Design review of the part built by this model. Coordinates are the model's own, in mm. Face numbers are marked on the shaded views. Coordinates: 2 decimals unless noted, no trailing zeros. Loops run counter-clockwise (first coordinate to the right, second up) from the corner with the lowest first, then second, coordinate; pieces in that order, holes last.
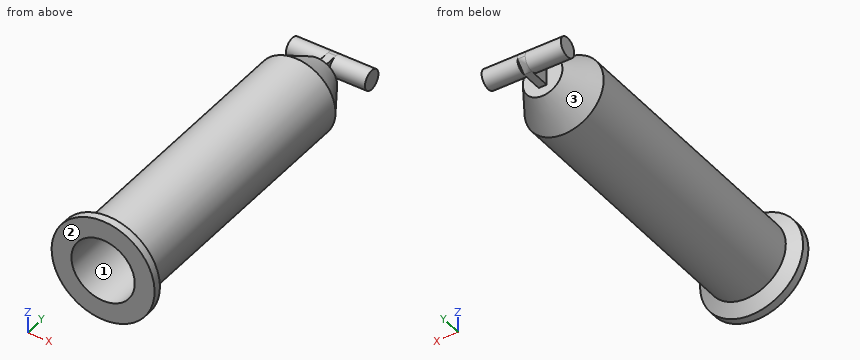
from build123d import *
from build123d.topology import SkipClean

# Parameters (mm, degrees)
SKETCH2_W                = 2
SKETCH2_H                = 5
BOSS_EXTRUDE1_DEPTH      = 8
CUT_EXTRUDE1_DEPTH       = 91.049986119
CUT_EXTRUDE1_DEPTH_BACK  = 91.049986119
SKETCH3_3_R              = 2.5
BOSS_EXTRUDE2_DEPTH      = 9
BOSS_EXTRUDE2_DEPTH_BACK = 11


with BuildPart() as part:
    # Sketch1 → Revolve1 (revolve)
    with BuildSketch(Plane(origin=(0, 0, 0), x_dir=(0, 0, -1), z_dir=(1, 0, 0))):
        Polygon((-10, 4), (-10, 72), (-5, 80), (0, 80), (0, 71.426407547), (-8, 71.426407547), (-8, 0), (-13, 0), (-13, 2), align=None)
    revolve(axis=Axis((0, 80, 0), (0, -1, 0)))

    # Sketch2 → Boss-Extrude1 (add)
    with BuildSketch(Plane(origin=(0, 80, 0), x_dir=(1, 0, 0), z_dir=(0, 1, 0))):
        Rectangle(SKETCH2_W, SKETCH2_H)
    extrude(amount=BOSS_EXTRUDE1_DEPTH)

    # Sketch3 → Cut-Extrude1 (cut, two sides)
    with BuildSketch(Plane.ZY.offset(1)) as cut_extrude1_sk:
        with BuildLine():
            ThreePointArc((-2.2e-08, 88), (1.767766945, 87.267766961), (2.5, 85.5))
            Line((2.5, 85.5), (2.5, 88))
            Line((2.5, 88), (-2.2e-08, 88))
        make_face()
        with BuildLine():
            Line((-2.5, 88), (-2.5, 85.5))
            ThreePointArc((-2.5, 85.5), (-1.767766961, 87.267766945), (-2.2e-08, 88))
            Line((-2.2e-08, 88), (-2.5, 88))
        make_face()
        Polygon((-2.5, 90.5), (-2.5, 88), (-2.2e-08, 88), (2.5, 88), (2.5, 90.5), align=None)
    extrude(amount=CUT_EXTRUDE1_DEPTH, mode=Mode.SUBTRACT)
    extrude(cut_extrude1_sk.sketch, amount=-CUT_EXTRUDE1_DEPTH_BACK, mode=Mode.SUBTRACT)

    # Sketch3_3 → Boss-Extrude2 (add, two sides)
    with SkipClean():  # the faces are left unmerged after this step: merging them gives an invalid solid
        with BuildSketch(Plane.ZY.offset(1)) as boss_extrude2_sk:
            with Locations((0, 85.5)):
                Circle(SKETCH3_3_R)
        extrude(amount=BOSS_EXTRUDE2_DEPTH)
        extrude(boss_extrude2_sk.sketch, amount=-BOSS_EXTRUDE2_DEPTH_BACK)


solid = part.part
Q1. Take a section at C-C, the plane y = 82. Write out the cut boundary in (x, z).
Q2. For line 1 (Z direction, x = 0, y = 36); line 2 (X direction, y = 61.5, z = -1.75), list the stretches that pass through material, from the lowest coordinate up.
Q3. Clearance check with flat-ended pins moving along their axes: pin 1 Ø4 at (y, z) = (85.5, 0.5) entering from -X; pin 2 Ø12 at (x, y) = (-9.5, 55) entering from +Z; pin 3 Ø4 at (x, y) = (-2.5, 67) entering from +Z. State where each tip first meets the part, or that it passes through.
Q4. Take a section at A-A, the plane x = 0. Write out the cut boundary in (y, z), then the cut area to 3 significant figures.
Q5. Take a section at B-B, the plane y = 53. Write out the cut boundary in (x, z), then the cut area to 3 significant figures.
Q6. The part is to be moulded in two halves that separate along X. For the marked faces 1, 2 and 3, say which applies: pulls with the +X half, pulls with the -X half, needs draft (parallel to the pull), parting line crosses it, or undercut.
Entries:
1. outline: (-1, -2.5) - (1, -2.5) - (1, 2.5) - (-1, 2.5) - close
2. line 1: z = -10 to -8, 8 to 10
2. line 2: x = -9.85 to -7.81, 7.81 to 9.85
3. pin 1: stops at x = -10
3. pin 2: stops at z = 9.37
3. pin 3: stops at z = 9.99
4. outline: (0, -13) - (2, -13) - (4, -10) - (72, -10) - (80, -5) - (80, -2.5) - (85.5, -2.5) arc R2.5 ccw to (85.5, 2.5) - (80, 2.5) - (80, 5) - (72, 10) - (4, 10) - (2, 13) - (0, 13) - (0, 8) - (71.43, 8) - (71.43, -8) - (0, -8) - close
4. area: 472 mm2
5. outline: circle Ø20 at (0, 0); hole circle Ø16 at (0, 0)
5. area: 113 mm2
6. face 1: undercut
6. face 2: needs draft
6. face 3: parting line crosses it
